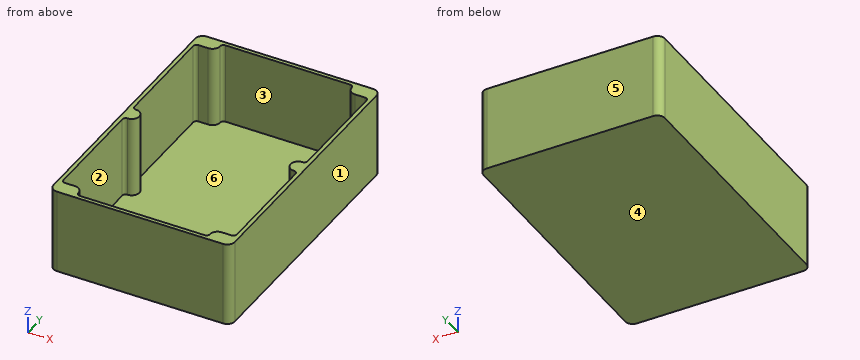
from build123d import *

# Parameters (mm, degrees)
F1_DEPTH = 3
F0_W     = 160
F0_H     = 240
F2_DEPTH = 74.8
F3_R     = 6.75
F4_R     = 2.99999


# Not quite as in the source:
# - a fillet or chamfer is up to 0.001 mm smaller than in the source, because OpenCascade refuses the exact size
# - ends of sketch curves that miss each other by under 0.0002 mm in the source are joined


with BuildPart() as f1:
    # F0 (on Top) → F1 (new body)
    with BuildSketch(Plane.XY):
        with BuildLine():
            Line((58.1, 113.45), (58.1, 116.5))
            Line((58.1, 116.5), (-58.1, 116.5))
            Line((-58.1, 116.5), (-58.1, 113.45))
            ThreePointArc((-58.1, 113.45), (-60.077029227, 108.677029227), (-64.85, 106.7))
            Line((-64.85, 106.7), (-76.5, 106.7))
            Line((-76.5, 106.7), (-76.5, 6.75))
            Line((-76.5, 6.75), (-73.5, 6.75))
            ThreePointArc((-73.5, 6.75), (-66.75, 0), (-73.5, -6.75))
            Line((-73.5, -6.75), (-76.5, -6.75))
            Line((-76.5, -6.75), (-76.5, -106.7))
            Line((-76.5, -106.7), (-64.7190213203, -106.7))
            ThreePointArc((-64.7190213203, -106.7), (-60.4393955388, -108.2301050614), (-58.1, -112.1267249867))
            Line((-58.1, -112.1267249867), (-58.1, -116.5))
            Line((-58.1, -116.5), (58.1, -116.5))
            Line((58.1, -116.5), (58.1, -113.45))
            ThreePointArc((58.1, -113.45), (60.077029227, -108.677029227), (64.85, -106.7))
            Line((64.85, -106.7), (76.5, -106.7))
            Line((76.5, -106.7), (76.5, -6.75))
            Line((76.5, -6.75), (73.5, -6.75))
            ThreePointArc((73.5, -6.75), (66.75, 0), (73.5, 6.75))
            Line((73.5, 6.75), (76.5, 6.75))
            Line((76.5, 6.75), (76.5, 106.7))
            Line((76.5, 106.7), (64.85, 106.7))
            ThreePointArc((64.85, 106.7), (60.077029227, 108.677029227), (58.1, 113.45))
        make_face()
    extrude(amount=F1_DEPTH)

    # F0 (on Top) → F2 (join)
    with BuildSketch(Plane.XY):
        Rectangle(F0_W, F0_H)
        Polygon((58.1, 116.5), (76.5, 116.5), (76.5, 106.7), (76.5, 6.75), (76.5, -6.75), (76.5, -106.7), (76.5, -116.5), (58.1, -116.5), (-58.1, -116.5), (-76.5, -116.5), (-76.5, -106.7), (-76.5, -6.75), (-76.5, 6.75), (-76.5, 106.7), (-76.5, 116.5), (-58.1, 116.5), align=None, mode=Mode.SUBTRACT)
        with BuildLine():
            Line((-58.1, 113.45), (-58.1, 116.5))
            Line((-58.1, 116.5), (-76.5, 116.5))
            Line((-76.5, 116.5), (-76.5, 106.7))
            Line((-76.5, 106.7), (-64.85, 106.7))
            ThreePointArc((-64.85, 106.7), (-60.077029227, 108.677029227), (-58.1, 113.45))
        make_face()
        with BuildLine():
            Line((76.5, 106.7), (76.5, 116.5))
            Line((76.5, 116.5), (58.1, 116.5))
            Line((58.1, 116.5), (58.1, 113.45))
            ThreePointArc((58.1, 113.45), (60.077029227, 108.677029227), (64.85, 106.7))
            Line((64.85, 106.7), (76.5, 106.7))
        make_face()
        with BuildLine():
            Line((-73.5, 6.75), (-76.5, 6.75))
            Line((-76.5, 6.75), (-76.5, -6.75))
            Line((-76.5, -6.75), (-73.5, -6.75))
            ThreePointArc((-73.5, -6.75), (-66.75, 0), (-73.5, 6.75))
        make_face()
        with BuildLine():
            Line((76.5, -6.75), (76.5, 6.75))
            Line((76.5, 6.75), (73.5, 6.75))
            ThreePointArc((73.5, 6.75), (66.75, 0), (73.5, -6.75))
            Line((73.5, -6.75), (76.5, -6.75))
        make_face()
        with BuildLine():
            Line((-64.7190213203, -106.7), (-76.5, -106.7))
            Line((-76.5, -106.7), (-76.5, -116.5))
            Line((-76.5, -116.5), (-58.1, -116.5))
            Line((-58.1, -116.5), (-58.1, -112.1267249867))
            ThreePointArc((-58.1, -112.1267249867), (-60.4393955388, -108.2301050614), (-64.7190213203, -106.7))
        make_face()
        with BuildLine():
            Line((76.5, -116.5), (76.5, -106.7))
            Line((76.5, -106.7), (64.85, -106.7))
            ThreePointArc((64.85, -106.7), (60.077029227, -108.677029227), (58.1, -113.45))
            Line((58.1, -113.45), (58.1, -116.500006485))
            Line((58.1, -116.500006485), (76.5, -116.5))
        make_face()
    extrude(amount=F2_DEPTH)

    # F3
    f3_edges = [f1.edges().sort_by_distance(p)[0] for p in [
        (80, 120, 37.4),
        (-80, 120, 37.4),
        (-80, -120, 37.4),
        (80, -120, 37.4),
    ]]
    fillet(f3_edges, radius=F3_R)

    # F4 (radius 3 in the source; OpenCascade refuses exactly that, so slightly less here)
    f4_edges = [f1.edges().sort_by_distance(p)[0] for p in [
        (-76.5, 106.7, 38.9),
        (-58.1, 116.5, 38.9),
        (-76.5, -6.75, 38.9),
        (58.1, 116.5, 38.9),
        (76.5, 106.7, 38.9),
        (76.5, -6.75, 38.9),
        (-76.5, 6.75, 38.9),
        (-76.5, -106.7, 38.9),
        (-58.1, -116.5, 38.9),
        (76.5, 6.75, 38.9),
        (76.5, -106.7, 38.9),
        (58.1, -116.5, 38.9),
    ]]
    fillet(f4_edges, radius=F4_R)


solid = f1.part
CAD build for the part. Positions are in the model's coordinates, mm. Face numbers are marked on the shaded views. A direction names the side the tool comes from. Coordinates: 2 decimals unless noted, no trailing zeros. Write each loop counter-clockwise with the first axis right and the second up, starting at its lowest first coordinate (ties: lowest second). Pieces come first, ordered by that corner, then holes. Notation, with made-up numbers: (41, -23) - (79, -23) arc R20 ccw to (79, -3) - close; hole circle Ø9 at (82.5, -15). An arc over 180 degrees is marked (long way). Use a Markdown table: item, result. Add a question column.
Item 1: Mould opens along X. For the marked faces 1, 2, 3 and 4 say: pulls with the +X half, pulls with the -X half, needs draft (parallel to the pull), parting line crosses it, or undercut.
Item 2: Drill centre lines: L1, parallel to Y at x = -73, z = 69; L2, parallel to X at y = -11.5, z = 63; L3, parallel to Y at x = 9, z = 62.5. Where is each one in solid material? Low to high. Write a range as from..to.
Item 3: Band-saw the part on B-B, the plane y = 0. Give the cut face in (x, z), and give its area (3 significant figures).
Item 4: 3-axis set-ups, long thin cutter, end or side, ignore diameter. For the marked faces 5 and 6: which of +Z, -Z, +X, -X, +Y, -Y reach the whole face in a straight line?
Item 5: Band-saw the part on A-A, the plane x = -4.5. Give the cut face in (y, z), and give its area (3 significant figures).
Item 6: Flat gauge pin, fed straight in: pin 1 (1.5 mm diameter, centred on x = -49.5, y = -53, fed in from +Z). Where does the tip first touch, or does it go through?
Numbers:
| question | item | result |
|---|---|---|
| 1 | face 1 | pulls with the +X half |
| 1 | face 2 | undercut |
| 1 | face 3 | undercut |
| 1 | face 4 | needs draft |
| 2 | L1 | -120..-106.7, -6.73..6.73, 106.7..120 |
| 2 | L2 | -80..-76.5, 76.5..80 |
| 2 | L3 | -120..-116.5, 116.5..120 |
| 3 | outline | (-80, 0) - (80, 0) - (80, 74.8) - (66.75, 74.8) - (66.75, 3) - (-66.75, 3) - (-66.75, 74.8) - (-80, 74.8) - close |
| 3 | area | 2,380 mm2 |
| 4 | face 5 | +Z, -Z, +X, -X, +Y |
| 4 | face 6 | +Z |
| 5 | outline | (-120, 0) - (120, 0) - (120, 74.8) - (116.5, 74.8) - (116.5, 3) - (-116.5, 3) - (-116.5, 74.8) - (-120, 74.8) - close |
| 5 | area | 1,220 mm2 |
| 6 | pin 1 | z = 3 |
